```python
from build123d import *

# Parameters (mm, degrees)
F1_DEPTH = 1.5875


with BuildPart() as f1:
    # F0 (on Top) → F1 (new body)
    with BuildSketch(Plane.XY):
        with BuildLine():
            Line((0, -44.45), (0, 44.45))
            ThreePointArc((0, 44.45), (-31.430896, 31.430896), (-44.45, 0))
            ThreePointArc((-44.45, 0), (-31.430896, -31.430896), (0, -44.45))
        make_face()
        with BuildLine():
            ThreePointArc((-28.575, 0), (-31.75, -3.175), (-34.925, 0))
            ThreePointArc((-34.925, 0), (-33.259902, 10.65526), (-28.423379, 20.294511))
            ThreePointArc((-28.423379, 20.294511), (-18.366773, 27.313204), (-23.54243, 16.195203))
            ThreePointArc((-23.54243, 16.195203), (-26.972249, 9.435487), (-28.504091, 2.011817))
            ThreePointArc((-28.504091, 2.011817), (-28.709383, 1.378157), (-28.565731, 0.727747))
            ThreePointArc((-28.565731, 0.727747), (-28.572683, 0.363903), (-28.575, 0))
        make_face(mode=Mode.SUBTRACT)
    extrude(amount=F1_DEPTH)


solid = f1.part
```
Can you work these out from the model? Positions are in its coordinate system, mm. A direction names the side the tool comes from. Coordinates: 2 decimals unless noted, no trailing zeros. Loops run counter-clockwise (first coordinate to the right, second up) from the corner with the lowest first, then second, coordinate; pieces in that order, holes last.
1) I need wall thicknesses on probe 1 along Y at (x, z) = (-25, 0.95); probe 2 along X at (y, z) = (16, 1); probe 3 along Y at (x, z) = (-23, 0.2). Which ranges of each line are inside material? Lowest first, please.
2) Imagine slicing it at C-C on x = -21. List the corners of the cut face in (y, z) for me.
3) Imagine slicing it at B-B on z = 0.8. List the corners of the cut face in (x, y) for me (3 decimals).
4) Imagine slicing it at A-A on x = -26.5. List the corners of the cut face in (y, z) for me, plus the area to 3 significant figures.
5) Thinking about a two-plate mould opening in X: for faces 3 (the cylindrical face through (-31.68, -3.174, 0.783)), 4 (the flat face through (-18, 1, 0)), 5 (the flat face through (0, -1, 1)), which applies, pulls with the +X half, pulls with the -X half, needs draft (parallel to the pull), parting line crosses it, or undercut?
6) Which directions (+Z, -Z, +X, -X, +Y, -Y) give clear straight access to the entire face, cutting with the end or side of a thin tool? Please do faces 1 (the cylindrical face through (-26.937, 9.536, 0.783)), 2 (the flat face through (-18, 1, 1.588)).
7) Imagine slicing it at D-D on y = -29. List the corners of the cut face in (x, z) for me.
Completed:
1. probe 1: y = -36.75 to 13.84, 28.27 to 36.75
1. probe 2: x = -41.47 to -31.04, -23.68 to 0
1. probe 3: y = -38.04 to 16.12, 28.78 to 38.04
2. outline: (-39.18, 0) - (16.27, 0) - (16.27, 1.59) - (-39.18, 1.59) - close; (28.63, 0) - (39.18, 0) - (39.18, 1.59) - (28.63, 1.59) - close
3. outline: (-44.45, 0) arc R44.45 ccw to (0, -44.45) - (0, 44.45) arc R44.45 ccw to start; hole (-34.925, 0) arc R3.175 ccw to (-28.575, 0) arc R28.57 cw to (-28.566, 0.728) arc R1.27 cw to (-28.504, 2.012) arc R28.575 cw to (-23.542, 16.195) arc R6.35 ccw (long way) to (-28.423, 20.295) arc R34.925 ccw to start
4. outline: (-35.69, 0) - (10.69, 0) - (10.69, 1.59) - (-35.69, 1.59) - close; (27.34, 0) - (35.69, 0) - (35.69, 1.59) - (27.34, 1.59) - close
4. area: 86.9 mm2
5. face 3: undercut
5. face 4: needs draft
5. face 5: pulls with the +X half
6. face 1: +Z, -Z
6. face 2: +Z, +X, -X, +Y, -Y
7. outline: (-33.69, 0) - (0, 0) - (0, 1.59) - (-33.69, 1.59) - close
